Could you check a few things on this model? Use its own coordinates, in mm. Coordinates: 2 decimals unless noted, no trailing zeros. Order: outer loops, then holes, each group sorted by start corner. A loop starts at its lowest first (then second) coordinate and runs counter-clockwise, first axis right, second up.
Autodesk Inventor part; units mm, degrees
ref_plane "YZ Plane" through (0, 0, 0) normal (1, 0, 0) x (0, 1, 0)
ref_plane "XZ Plane" through (0, 0, 0) normal (0, 1, 0) x (-1, 0, 0)
ref_plane "XY Plane" through (0, 0, 0) normal (0, 0, 1) x (1, 0, 0)
sketch "Sketch1" plane through (0, 0, 0) normal (1, 0, 0) x (0, 1, 0)
  line L0 (0, 0) -> (0, 355.6)
  line L1 (0, 355.6) -> (-50.8, 228.6)
  line L2 (-50.8, 228.6) -> (-203.2, 127)
  line L3 (-203.2, 127) -> (-685.8, 0)
  line L4 (-685.8, 0) -> (0, 0)
  dimension "d0" = 355.6
  dimension "d1" = 127
  dimension "d2" = 50.8
  dimension "d3" = 203.2
  dimension "d4" = 127
  dimension "d5" = 685.8
extrude "Extrusion1" add sketch "Sketch1" along normal blind 3.175
sketch "Sketch2" plane through (0, 0, 355.6) normal (0, 1, 0) x (1, 0, 0)
  line L0 (0, 355.6) -> (0, 0)
  line L1 (0, 0) -> (3.175, 0)
  line L2 (3.175, 355.6) -> (3.175, 0)
  line L3 (0, 355.6) -> (3.175, 355.6)
extrude "Extrusion2" add sketch "Sketch2" along normal blind 25.4
properties part number "15102898-16-P-0102" material "ABS Plastic"
Item 1: Suppose I cut it at A-A (x = 0.7). List the corners of the cut face in (y, z) for me, and give its area (3 significant figures).
Item 2: I need wall thicknesses on line 1 (Z direction, x = 0.2, y = -375.5); line 2 (Y direction, x = 1.9, z = 137); line 3 (Z direction, x = 2.3, y = -443.5). Which ranges of each line are inside material? Lowest first, please.
Item 3: Suppose I cut it at B-B (y = -36.5). List the corners of the cut face in (x, z) for me (3 decimals), and give its area (3 significant figures).
Item 4: Suppose I cut it at C-C (z = 293). List the corners of the cut face in (x, y) for me (3 decimals), and give its area (3 significant figures).
Geometry results:
1. outline: (-685.8, 0) - (25.4, 0) - (25.4, 355.6) - (0, 355.6) - (-50.8, 228.6) - (-203.2, 127) - close
1. area: 81,600 mm2
2. line 1: z = 0 to 81.66
2. line 2: y = -188.2 to 25.4
2. line 3: z = 0 to 63.76
3. outline: (0, 0) - (3.175, 0) - (3.175, 264.35) - (0, 264.35) - close
3. area: 839 mm2
4. outline: (0, -25.04) - (3.175, -25.04) - (3.175, 25.4) - (0, 25.4) - close
4. area: 160 mm2
